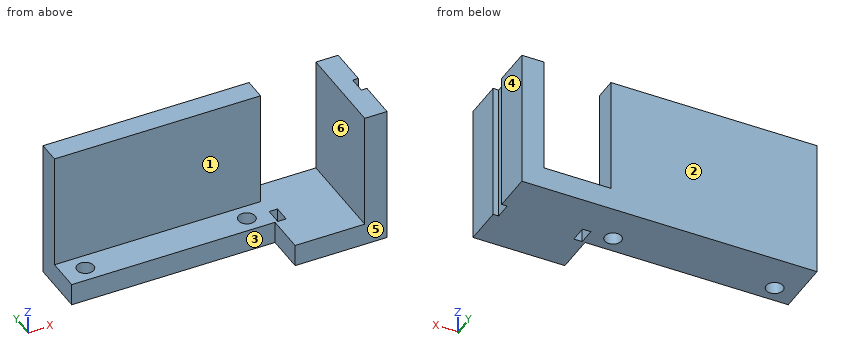
```python
from build123d import *

# Parameters (mm, degrees)
CROQUIS1_W              = 37
CROQUIS1_H              = 10
SALIENTE_EXTRUIR1_DEPTH = 25
CROQUIS2_W              = 37
CROQUIS2_H              = 6
CORTAR_EXTRUIR1_DEPTH   = 21
CROQUIS4_R              = 1.5
CORTAR_EXTRUIR2_DEPTH   = 4
CROQUIS5_W              = 4
CROQUIS5_H              = 10
SALIENTE_EXTRUIR2_DEPTH = 16
CROQUIS6_W              = 4
CROQUIS6_H              = 10
SALIENTE_EXTRUIR3_DEPTH = 21
CROQUIS7_W              = 1.5
CROQUIS7_H              = 3
CORTAR_EXTRUIR3_DEPTH   = 4
SALIENTE_EXTRUIR4_DEPTH = 7
CORTAR_EXTRUIR4_START   = -25
CROQUIS9_W              = 0.995479253
CROQUIS9_H              = 3
CORTAR_EXTRUIR4_DEPTH   = 25


with BuildPart() as part:
    # Croquis1 → Saliente-Extruir1 (new body)
    with BuildSketch(Plane.XY):
        with Locations((-18.845794393, 11.401869159)):
            Rectangle(CROQUIS1_W, CROQUIS1_H)
    extrude(amount=SALIENTE_EXTRUIR1_DEPTH)

    # Croquis2 → Cortar-Extruir1 (cut)
    with BuildSketch(Plane.XY.offset(25)):
        with Locations((-18.845794393, 9.401869159)):
            Rectangle(CROQUIS2_W, CROQUIS2_H)
    extrude(amount=-CORTAR_EXTRUIR1_DEPTH, mode=Mode.SUBTRACT)

    # Croquis4 → Cortar-Extruir2 (cut)
    with BuildSketch(Plane.XY.offset(4)):
        with Locations((-33.345794393, 9.401869159)):
            Circle(CROQUIS4_R)
        with Locations((-4.345794393, 9.401869159)):
            Circle(CROQUIS4_R)
    extrude(amount=-CORTAR_EXTRUIR2_DEPTH, mode=Mode.SUBTRACT)

    # Croquis5 → Saliente-Extruir2 (add)
    with BuildSketch(Plane(origin=(-0.345794393, 0, 0), x_dir=(0, 0, -1), z_dir=(1, 0, 0))):
        with Locations((-2, 11.401869159)):
            Rectangle(CROQUIS5_W, CROQUIS5_H)
    extrude(amount=SALIENTE_EXTRUIR2_DEPTH)

    # Croquis6 → Saliente-Extruir3 (add)
    with BuildSketch(Plane.XY.offset(4)):
        with Locations((13.654205607, 11.401869159)):
            Rectangle(CROQUIS6_W, CROQUIS6_H)
    extrude(amount=SALIENTE_EXTRUIR3_DEPTH)

    # Croquis7 → Cortar-Extruir3 (cut)
    with BuildSketch(Plane.XY.offset(4)):
        with Locations((0.404205607, 7.901869159)):
            Rectangle(CROQUIS7_W, CROQUIS7_H)
    extrude(amount=-CORTAR_EXTRUIR3_DEPTH, mode=Mode.SUBTRACT)

    # Croquis8 → Saliente-Extruir4 (add)
    with BuildSketch(Plane.XZ.offset(-6.401869159)):
        Polygon((11.654205607, 25), (15.654205607, 25), (15.654205607, 0), (-0.845794393, 0), (-0.845794393, 4), (11.654205607, 4), align=None)
    extrude(amount=SALIENTE_EXTRUIR4_DEPTH)

    # Croquis9 → Cortar-Extruir4 (cut)
    with BuildSketch(Plane(origin=(0, 0, 0), x_dir=(-1, 0, 0), z_dir=(0, 0, -1)).offset(CORTAR_EXTRUIR4_START)):
        with Locations((-15.156465981, 7.901869159)):
            Rectangle(CROQUIS9_W, CROQUIS9_H)
    extrude(amount=CORTAR_EXTRUIR4_DEPTH, mode=Mode.SUBTRACT)


solid = part.part
```
Verification items for the finished model (mm, model axes). Face numbers are marked on the shaded views. A direction names the side the tool comes from. Round coordinates to 2 decimals unless told otherwise and drop trailing zeros. Write each loop counter-clockwise with the first axis right and the second up, starting at its lowest first coordinate (ties: lowest second). Pieces come first, ordered by that corner, then holes.
1. Access from +Z, -Z, +X, -X, +Y, -Y to the whole of each face (thin tool, end or side, straight path). Record for the marked faces 1, 2 and 3.
2. Draft check along X on the marked faces 4, 5 and 6. Enter one of: +X half, -X half, draft (parallel to the pull), parting line (faces both ways), or undercut.
3. Scan lines: L1, parallel to X at y = 6.75, z = 1; L2, parallel to X at y = 14.25, z = 20.25; L3, parallel to Z at x = -20.5, y = 9. Record each from-to range of solid material in increasing order.
4. Section check A-A on z = 2.75. Enter the section's corners in (x, y).
5. Gauge pin test, flat ends, axial feed: P1, Ø1.2, axis at x = -19, z = 2, coming from the -Y side; P2, Ø3, axis at x = -8.5, y = 13.5, coming from the -Z side; P3, Ø5, axis at x = -33.35, y = 9.4, coming from the +Z side; P4, Ø6, axis at x = -4, z = 14, coming from the -Y side. Record the tip position at first contact, or that the pin passes through.
6. Section check D-D on y = 8.5. Enter the section's corners in (x, z).
7. Section check C-C on x = -30.5. Enter the section's corners in (y, z), plus the area to 3 significant figures.
8. Section check B-B on z = 14. Enter the section's corners in (x, y).
Answer:
1. face 1: +Z, -X, -Y
1. face 2: +Z, -Z, +X, -X, +Y
1. face 3: +Z, -Z, -X, -Y
2. face 4: +X half
2. face 5: draft
2. face 6: undercut
3. L1: x = -37.35 to -0.35, 1.15 to 14.66
3. L2: x = -37.35 to -0.35, 11.65 to 15.65
3. L3: z = 0 to 4
4. outline: (-37.35, 6.4) - (-0.85, 6.4) - (-0.85, -0.6) - (15.65, -0.6) - (15.65, 6.4) - (14.66, 6.4) - (14.66, 9.4) - (15.65, 9.4) - (15.65, 16.4) - (-37.35, 16.4) - close; hole circle Ø3 at (-33.35, 9.4); hole circle Ø3 at (-4.35, 9.4); hole (-0.35, 6.4) - (1.15, 6.4) - (1.15, 9.4) - (-0.35, 9.4) - close
5. P1: stops at y = 6.4
5. P2: stops at z = 0
5. P3: stops at z = 4
5. P4: stops at y = 12.4
6. outline: (-37.35, 0) - (-34.54, 0) - (-34.54, 4) - (-37.35, 4) - close; (-32.15, 0) - (-5.54, 0) - (-5.54, 4) - (-32.15, 4) - close; (-3.15, 0) - (-0.35, 0) - (-0.35, 4) - (-3.15, 4) - close; (1.15, 0) - (14.66, 0) - (14.66, 25) - (11.65, 25) - (11.65, 4) - (1.15, 4) - close
7. outline: (6.4, 0) - (16.4, 0) - (16.4, 25) - (12.4, 25) - (12.4, 4) - (6.4, 4) - close
7. area: 124 mm2
8. outline: (-37.35, 12.4) - (-0.35, 12.4) - (-0.35, 16.4) - (-37.35, 16.4) - close; (11.65, -0.6) - (15.65, -0.6) - (15.65, 6.4) - (14.66, 6.4) - (14.66, 9.4) - (15.65, 9.4) - (15.65, 16.4) - (11.65, 16.4) - close
